Source: CAD feature listing. Evaluate the final solid. Frame: model axes, mm. A direction names the side the tool comes from. Give positions to 0.01 mm unless a question says otherwise; leave off trailing zeros. Write each loop counter-clockwise with the first axis right and the second up, starting at its lowest first coordinate (ties: lowest second). Pieces come first, ordered by that corner, then holes. Notation, with made-up numbers: (67.25, -14.75) -> (117.25, -14.75) arc R15 ccw to (117.25, -10.75) -> close; hole circle Ø5 at (18.25, 62.5). An arc over 180 degrees is marked (long way). Answer as a JSON object with one key per item and string values. Group by question number.
Item 1: Pull-direction query (Y, two-part tool) for faces 1 (the face through (0, 0, 6)), 2 (the face through (1.6, 5.7, 0.75)); classes: pulls with the +Y half, pulls with the -Y half, needs draft (parallel to the pull), parting line crosses it, or undercut.
Item 2: Section query A-A on y = 0. Return the cut outline in (x, z), plus the area to 3 significant figures.
Item 3: First-contact query: pin 1 Ø1 at (x, y) = (-0.5, 4.5) entering from -Z; pin 2 Ø1 at (y, z) = (3, -4) entering from +X. Flat tips, straight axial feed; report the tip coordinate or a pass-through.
Item 4: Ray query, probe 1 along Y at (x, z) = (1.6, 0); probe 2 along Y at (x, z) = (-1.5, -2.25); probe 3 along Z at (x, y) = (1.6, 2.5). Return the intervals inside material, ascending. Write a range as from..to.
Item 5: Access query for faces 3 (the face through (1.6, -2.59, 3.37)), 4 (the face through (-1.6, -2.59, 3.37)), 5 (the face through (0.024, -3.905, 0.867)). Directions: +Z, -Z, +X, -X, +Y, -Y. A direction counts if a zero-diameter tool reaches every point of the face in a straight line with its end or side. Return the directions, or none.
Item 6: Section query D-D on z = 4.5. Return the cut outline in (x, y), plus the area to 3 significant figures.
Item 7: Section query C-C on x = 0.65. Return the cut outline in (y, z), plus the area to 3 significant figures.
from build123d import *

# Parameters (mm, degrees)
SKETCH1_R           = 6
BOSS_EXTRUDE1_DEPTH = 1.75
CUT_EXTRUDE1_REACH  = 11.179
SKETCH2_R           = 4
SKETCH3_R           = 5.75
SKETCH3_R_2         = 4.25
CUT_EXTRUDE2_DEPTH  = 0.3


with BuildPart() as part:
    # Sketch1 → Boss-Extrude1 (new, symmetric)
    with BuildSketch(Plane(origin=(0, 0, 0), x_dir=(0, 0, -1), z_dir=(1, 0, 0))):
        Circle(SKETCH1_R)
    extrude(amount=BOSS_EXTRUDE1_DEPTH, both=True)

    # Sketch2 → Cut-Extrude1 (cut, up to next)
    with BuildSketch(Plane(origin=(1.75, 0, 0), x_dir=(0, 0, -1), z_dir=(1, 0, 0)), mode=Mode.PRIVATE) as cut_extrude1_sk1:
        Circle(SKETCH2_R)
    cut_extrude1_tool1 = extrude(cut_extrude1_sk1.sketch, amount=-CUT_EXTRUDE1_REACH, mode=Mode.PRIVATE) & part.part
    add(cut_extrude1_tool1.solids().sort_by_distance((1.75, 0, 0))[0], mode=Mode.SUBTRACT)

    # Sketch3 → Cut-Extrude2 (cut)
    with BuildSketch(Plane(origin=(1.75, 0, 0), x_dir=(0, 0, -1), z_dir=(1, 0, 0))):
        Circle(SKETCH3_R)
        Circle(SKETCH3_R_2, mode=Mode.SUBTRACT)
    cut_extrude2 = extrude(amount=-CUT_EXTRUDE2_DEPTH, mode=Mode.SUBTRACT)

    # Mirror1: Cut-Extrude2 across plane
    add(cut_extrude2.mirror(Plane(origin=(0, 0, 0), x_dir=(0, 0, 1), z_dir=(1, 0, 0))), mode=Mode.SUBTRACT)


solid = part.part
Worked answers:
{
 "1": {"face 1": "parting line crosses it", "face 2": "undercut"},
 "2": {"outline": "(-1.75, -6) -> (1.75, -6) -> (1.75, -5.75) -> (1.45, -5.75) -> (1.45, -4.25) -> (1.75, -4.25) -> (1.75, -4) -> (-1.75, -4) -> (-1.75, -4.25) -> (-1.45, -4.25) -> (-1.45, -5.75) -> (-1.75, -5.75) -> close; (-1.75, 4) -> (1.75, 4) -> (1.75, 4.25) -> (1.45, 4.25) -> (1.45, 5.75) -> (1.75, 5.75) -> (1.75, 6) -> (-1.75, 6) -> (-1.75, 5.75) -> (-1.45, 5.75) -> (-1.45, 4.25) -> (-1.75, 4.25) -> close", "area": "12.2 mm^2"},
 "3": {"pin 1": "z = -4.47", "pin 2": "x = 1.45"},
 "4": {"probe 1": "-6..-5.75, -4.25..-4, 4..4.25, 5.75..6", "probe 2": "-5.56..-5.29, -3.61..-3.31, 3.31..3.61, 5.29..5.56", "probe 3": "-5.45..-5.18, -3.44..-3.12, 3.12..3.44, 5.18..5.45"},
 "5": {"face 3": "+X", "face 4": "-X", "face 5": "+X, -X"},
 "6": {"outline": "(-1.75, -3.97) -> (1.75, -3.97) -> (1.75, -3.58) -> (1.45, -3.58) -> (1.45, 3.58) -> (1.75, 3.58) -> (1.75, 3.97) -> (-1.75, 3.97) -> (-1.75, 3.58) -> (-1.45, 3.58) -> (-1.45, -3.58) -> (-1.75, -3.58) -> close", "area": "23.5 mm^2"},
 "7": {"outline": "circle Ø12 at (0, 0); hole circle Ø8 at (0, 0)", "area": "62.8 mm^2"}
}
